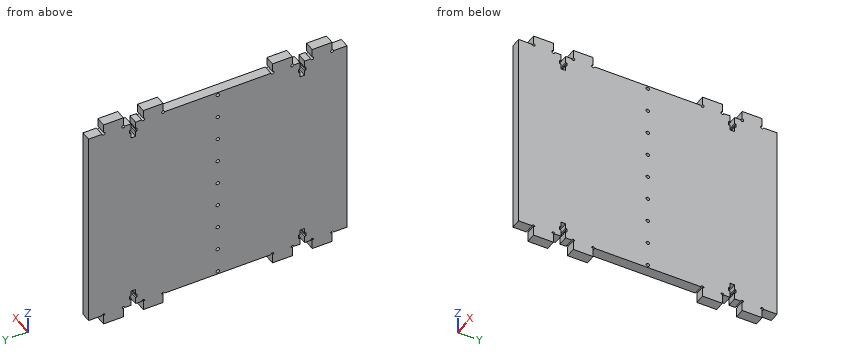
from build123d import *

# Parameters (mm, degrees)
SKETCH1_W                = 206
SKETCH1_H                = 260
EXTRUDE1_DEPTH           = 10
SKETCH3_W                = 10
SKETCH3_H                = 20
EXTRUDE2_DEPTH           = 10
LPATTERN1_COUNT          = 2
LPATTERN1_PITCH          = 196
LPATTERN1_COUNT_DIR2     = 2
LPATTERN1_PITCH_DIR2     = 170
EXTRUDE4_DEPTH           = 10
LPATTERN2_COUNT          = 2
LPATTERN2_PITCH          = 170
LPATTERN2_COPY_1_DEPTH   = 10
EXTRUDE5_DEPTH           = 10
MIRROR3_COPY_1_DEPTH     = 10
M3_CLEARANCE_HOLE1_D     = 3.4
M3_CLEARANCE_HOLE1_DEPTH = 10
M3_CLEARANCE_HOLE1_TIP   = 1.021463052
MIRROR4_COPY_1_SKETCH_W  = 10
MIRROR4_COPY_1_SKETCH_H  = 20
MIRROR4_COPY_1_DEPTH     = 10


with BuildPart() as part:
    # Sketch1 → Extrude1 (new body)
    with BuildSketch(Plane(origin=(0, 0, 0), x_dir=(0, 0, -1), z_dir=(1, 0, 0))):
        Rectangle(SKETCH1_W, SKETCH1_H)
    extrude(amount=EXTRUDE1_DEPTH)

    # Sketch3 → Extrude2 (add)
    with BuildSketch(Plane(origin=(10, 0, 0), x_dir=(0, 0, -1), z_dir=(1, 0, 0))):
        with Locations((-108, -105)):
            Rectangle(SKETCH3_W, SKETCH3_H)
        with Locations((-108, -65)):
            Rectangle(SKETCH3_W, SKETCH3_H)
    extrude2 = extrude(amount=-EXTRUDE2_DEPTH)

    # LPattern1: Extrude2 2 × 2, 2 skipped
    with Locations(*[(i * LPATTERN1_PITCH, j * LPATTERN1_PITCH_DIR2, 0) for i in range(LPATTERN1_COUNT) for j in range(LPATTERN1_COUNT_DIR2) if (i, j) not in ((0, 0), (1, 0), (1, 1))]):
        add(extrude2)

    # Sketch5 → Extrude4 (cut)
    with BuildSketch(Plane(origin=(10, 0, 0), x_dir=(0, 0, -1), z_dir=(1, 0, 0))):
        Polygon((-103, -87.25), (-96, -87.25), (-96, -88.625), (-92.3, -88.625), (-92.3, -87.25), (-87, -87.25), (-87, -82.75), (-92.3, -82.75), (-92.3, -81.375), (-96, -81.375), (-96, -82.75), (-103, -82.75), align=None)
    extrude4 = extrude(amount=-EXTRUDE4_DEPTH, mode=Mode.SUBTRACT)

    # Mirror1: Extrude4 across plane
    add(extrude4.mirror(Plane(origin=(0, 0, 0), x_dir=(1, 0, 0), z_dir=(0, 0, -1))), mode=Mode.SUBTRACT)

    # LPattern2: Extrude4 ×2
    with Locations(*[(0, i * LPATTERN2_PITCH, 0) for i in range(1, LPATTERN2_COUNT)]):
        add(extrude4, mode=Mode.SUBTRACT)

    # LPattern2 copy 1 sketch → LPattern2 copy 1 (cut)
    with BuildSketch(Plane(origin=(10, 170, 0), x_dir=(0, 0, 1), z_dir=(1, 0, 0))):
        Polygon((-103, 87.25), (-96, 87.25), (-96, 88.625), (-92.3, 88.625), (-92.3, 87.25), (-87, 87.25), (-87, 82.75), (-92.3, 82.75), (-92.3, 81.375), (-96, 81.375), (-96, 82.75), (-103, 82.75), align=None)
    extrude(amount=-LPATTERN2_COPY_1_DEPTH, mode=Mode.SUBTRACT)

    # Sketch6 → Extrude5 (cut)
    with BuildSketch(Plane(origin=(10, 0, 0), x_dir=(0, 0, -1), z_dir=(1, 0, 0))):
        with BuildLine():
            Line((-104.5, -115), (-103, -115))
            Line((-103, -115), (-103, -116.5))
            ThreePointArc((-103, -116.5), (-101.939339828, -113.939339828), (-104.5, -115))
        make_face()
        with BuildLine():
            Line((-104.5, -55), (-103, -55))
            Line((-103, -55), (-103, -53.5))
            ThreePointArc((-103, -53.5), (-101.939339828, -56.060660172), (-104.5, -55))
        make_face()
        with BuildLine():
            Line((-104.5, -95), (-103, -95))
            Line((-103, -95), (-103, -93.5))
            ThreePointArc((-103, -93.5), (-101.939339828, -96.060660172), (-104.5, -95))
        make_face()
        with BuildLine():
            Line((-104.5, -75), (-103, -75))
            Line((-103, -75), (-103, -76.5))
            ThreePointArc((-103, -76.5), (-101.939339828, -73.939339828), (-104.5, -75))
        make_face()
    extrude5 = extrude(amount=-EXTRUDE5_DEPTH, mode=Mode.SUBTRACT)

    # Mirror2: Extrude5 across plane
    add(extrude5.mirror(Plane(origin=(0, 0, 0), x_dir=(1, 0, 0), z_dir=(0, 0, -1))), mode=Mode.SUBTRACT)

    # Mirror3: Extrude5 across plane
    add(extrude5.mirror(Plane.ZX), mode=Mode.SUBTRACT)

    # Mirror3 copy 1 sketch → Mirror3 copy 1 (cut)
    with BuildSketch(Plane(origin=(10, 0, 0), x_dir=(0, 0, 1), z_dir=(1, 0, 0))):
        with BuildLine():
            Line((-104.5, -115), (-103, -115))
            Line((-103, -115), (-103, -116.5))
            ThreePointArc((-103, -116.5), (-101.939339828, -113.939339828), (-104.5, -115))
        make_face()
        with BuildLine():
            Line((-104.5, -55), (-103, -55))
            Line((-103, -55), (-103, -53.5))
            ThreePointArc((-103, -53.5), (-101.939339828, -56.060660172), (-104.5, -55))
        make_face()
        with BuildLine():
            Line((-104.5, -95), (-103, -95))
            Line((-103, -95), (-103, -93.5))
            ThreePointArc((-103, -93.5), (-101.939339828, -96.060660172), (-104.5, -95))
        make_face()
        with BuildLine():
            Line((-104.5, -75), (-103, -75))
            Line((-103, -75), (-103, -76.5))
            ThreePointArc((-103, -76.5), (-101.939339828, -73.939339828), (-104.5, -75))
        make_face()
    extrude(amount=-MIRROR3_COPY_1_DEPTH, mode=Mode.SUBTRACT)

    # M3 Clearance Hole1
    with Locations(Plane(origin=(10, -130, 293), x_dir=(0, -1, 0), z_dir=(1, 0, 0))):
        with Locations((-130, 368), (-130, 343), (-130, 318), (-130, 293), (-130, 268), (-130, 243), (-130, 218), (-130, 193), (-130, 393)):
            Hole(M3_CLEARANCE_HOLE1_D / 2, depth=M3_CLEARANCE_HOLE1_DEPTH)
            with Locations((0, 0, -(M3_CLEARANCE_HOLE1_DEPTH + M3_CLEARANCE_HOLE1_TIP / 2))):  # 118° drill point
                Cone(0, M3_CLEARANCE_HOLE1_D / 2, M3_CLEARANCE_HOLE1_TIP, mode=Mode.SUBTRACT)

    # Mirror4: Extrude2 across plane
    add(extrude2.mirror(Plane(origin=(0, 0, 0), x_dir=(1, 0, 0), z_dir=(0, 0, -1))))

    # Mirror4 copy 1 sketch → Mirror4 copy 1 (add)
    with BuildSketch(Plane(origin=(10, 170, 0), x_dir=(0, 0, 1), z_dir=(1, 0, 0))):
        with Locations((-108, 105)):
            Rectangle(MIRROR4_COPY_1_SKETCH_W, MIRROR4_COPY_1_SKETCH_H)
        with Locations((-108, 65)):
            Rectangle(MIRROR4_COPY_1_SKETCH_W, MIRROR4_COPY_1_SKETCH_H)
    extrude(amount=-MIRROR4_COPY_1_DEPTH)


solid = part.part
Design review of the part built by this model. Coordinates are the model's own, in mm. Coordinates: 2 decimals unless noted, no trailing zeros. Order: outer loops, then holes, each group sorted by start corner. A loop starts at its lowest first (then second) coordinate and runs counter-clockwise, first axis right, second up. Notation, with made-up numbers: (-11, 48) -> (16, 48) arc R22 ccw to (16, 84) -> close; hole circle Ø9 at (38, -15). An arc over 180 degrees is marked (long way). One line per item, written item: value.
1) We need section A-A, the plane x = 7.75. Count the separate pieces of the cut face and the enclosed holes in it, then the cut area to 3 significant figures.
Output values:
separate pieces: 1
enclosed holes: 9
area: 54,700 mm2
2) To check wall thickness, follow probe 1 along Y at (x, z) = (7, -103.5); probe 2 along Y at (x, z) = (5, -100); probe 3 along Y at (x, z) = (4.5, 75). State the ranges of each line that lie inside material, in increasing order. Write a range as [from, to].
Output values:
probe 1: y = [-115, -95], [-75, -55], [55, 75], [95, 115]
probe 2: y = [-130, -87.25], [-82.75, -1.7], [1.7, 82.75], [87.25, 130]
probe 3: y = [-130, -1.7], [1.7, 130]
3) Clearance check with flat-ended pins moving along their axes: P1, Ø1.9, axis at x = 5, y = -80, coming from the +Z side; P2, Ø1.5, axis at x = 2.5, y = 82, coming from the -Z side; P3, Ø1.5, axis at y = 44.5, z = -8.5, coming from the -X side; P4, Ø2, axis at x = 5.5, y = -86, coming from the +Z side. State where each tip first meets the part, or that it passes through.
Output values:
P1: stops at z = 103
P2: stops at z = -103
P3: stops at x = 0
P4: stops at z = 87
4) We need section B-B, the plane y = -49.5. Give the boundary of the cut face in (x, z), then the cut area to 3 significant figures.
Output values:
outline: (0, -103) -> (10, -103) -> (10, 103) -> (0, 103) -> close
area: 2,060 mm2
